Build history of the part. All positions in model axes, mm. Face numbers are marked on the shaded views. Round coordinates to 2 decimals unless told otherwise and drop trailing zeros. Order: outer loops, then holes, each group sorted by start corner. A loop starts at its lowest first (then second) coordinate and runs counter-clockwise, first axis right, second up. Notation, with made-up numbers: (76, 54) -> (118, 54) arc R34 cw to (118, 92) -> close; hole circle Ø8 at (67, 51). An arc over 180 degrees is marked (long way). Answer as a JSON object with one key per item and string values.
from build123d import *

# Parameters (mm, degrees)
BOSS_EXTRUDE1_DEPTH = 4
SKETCH2_R           = 6
BOSS_EXTRUDE2_DEPTH = 1
SKETCH3_R           = 3.95
BOSS_EXTRUDE3_DEPTH = 7
SKETCH4_R           = 2
CUT_EXTRUDE1_DEPTH  = 113.187343315


with BuildPart() as part:
    # Sketch1 → Boss-Extrude1 (new body)
    with BuildSketch(Plane(origin=(0, 0, 0), x_dir=(1, 0, 0), z_dir=(0, 1, 0))):
        with BuildLine():
            Line((0, 11), (100, 11))
            ThreePointArc((100, 11), (111, 0), (100, -11))
            Line((100, -11), (0, -11))
            ThreePointArc((0, -11), (-11, 0), (0, 11))
        make_face()
    extrude(amount=BOSS_EXTRUDE1_DEPTH)

    # Sketch2 → Boss-Extrude2 (add)
    with BuildSketch(Plane(origin=(0, 4, 0), x_dir=(1, 0, 0), z_dir=(0, 1, 0))):
        with Locations(Location((0, 0, 0), (0, 0, 270))):
            Circle(SKETCH2_R)
        with Locations(Location((100, 0, 0), (0, 0, 270))):
            Circle(SKETCH2_R)
    extrude(amount=BOSS_EXTRUDE2_DEPTH)

    # Sketch3 → Boss-Extrude3 (add)
    with BuildSketch(Plane(origin=(0, 5, 0), x_dir=(1, 0, 0), z_dir=(0, 1, 0))):
        with Locations(Location((0, 0, 0), (0, 0, 270))):
            Circle(SKETCH3_R)
        with Locations(Location((100, 0, 0), (0, 0, 270))):
            Circle(SKETCH3_R)
    extrude(amount=BOSS_EXTRUDE3_DEPTH)

    # Sketch4 → Cut-Extrude1 (cut, through all)
    with BuildSketch(Plane(origin=(0, 12, 0), x_dir=(1, 0, 0), z_dir=(0, 1, 0))):
        with Locations(Location((0, 0, 0), (0, 0, 270))):
            Circle(SKETCH4_R)
        with Locations(Location((100, 0, 0), (0, 0, 270))):
            Circle(SKETCH4_R)
    extrude(amount=-CUT_EXTRUDE1_DEPTH, mode=Mode.SUBTRACT)


solid = part.part
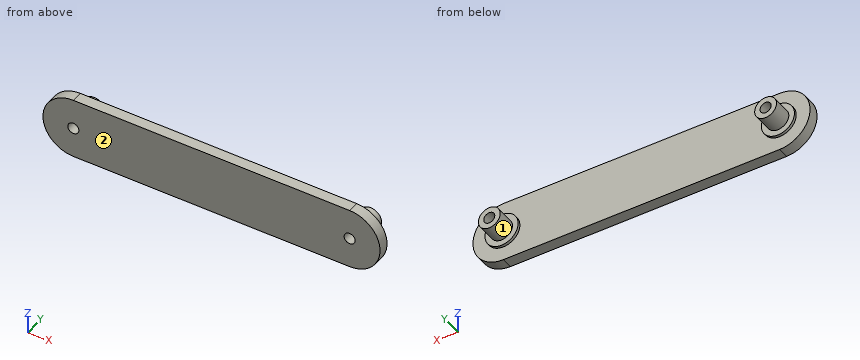
1) Pull direction X, two halves, no side cores. Call the marked faces 1 and 2: pulls with the +X half, pulls with the -X half, needs draft (parallel to the pull), parting line crosses it, or undercut.
Checked values:
{"face 1": "undercut", "face 2": "needs draft"}
2) Cut at C-C, the plane y = 2. Give the cut face in (x, z).
Checked values:
{"outline": "(0, -11) -> (100, -11) arc R11 ccw to (100, 11) -> (0, 11) arc R11 ccw to start; hole circle Ø4 at (0, 0); hole circle Ø4 at (100, 0)"}
3) Flat gauge pins, fed straight in: pin 1 Ø6.5 at (x, z) = (78.5, 4.5) entering from +Y; pin 2 Ø2 at (y, z) = (3.5, -7.5) entering from +X; pin 3 Ø5 at (y, z) = (8.5, -6) entering from -X. Where does each tip first touch, or does it go through?
Checked values:
{"pin 1": "stops at y = 4", "pin 2": "stops at x = 108.87", "pin 3": "stops at x = -1.83"}
4) Cut at A-A, the plane z = 0. Give the cut face in (x, y), plus the area to 3 significant figures.
Checked values:
{"outline": "(-11, 0) -> (-2, 0) -> (-2, 12) -> (-3.95, 12) -> (-3.95, 5) -> (-6, 5) -> (-6, 4) -> (-11, 4) -> close; (2, 0) -> (98, 0) -> (98, 12) -> (96.05, 12) -> (96.05, 5) -> (94, 5) -> (94, 4) -> (6, 4) -> (6, 5) -> (3.95, 5) -> (3.95, 12) -> (2, 12) -> close; (102, 0) -> (111, 0) -> (111, 4) -> (106, 4) -> (106, 5) -> (103.95, 5) -> (103.95, 12) -> (102, 12) -> close", "area": "527 mm²"}
5) Probe L1, parallel to X at y = 3, z = 0; L2, parallel to X at y = 5.75, z = 0; L3, parallel to X at y = 4.75, z = 0. List the from-to ranges inside material, lowest first. Write a range as from..to.
Checked values:
{"L1": "x = -11..-2, 2..98, 102..111", "L2": "x = -3.95..-2, 2..3.95, 96.05..98, 102..103.95", "L3": "x = -6..-2, 2..6, 94..98, 102..106"}
6) Cut at B-B, the plane y = 9. Give the cut face in (x, z).
Checked values:
{"outline": "circle Ø7.9 at (0, 0); circle Ø7.9 at (100, 0); hole circle Ø4 at (0, 0); hole circle Ø4 at (100, 0)"}
7) Cut at D-D, the plane z = 5. Give the cut face in (x, y).
Checked values:
{"outline": "(-9.8, 0) -> (109.8, 0) -> (109.8, 4) -> (103.32, 4) -> (103.32, 5) -> (96.68, 5) -> (96.68, 4) -> (3.32, 4) -> (3.32, 5) -> (-3.32, 5) -> (-3.32, 4) -> (-9.8, 4) -> close"}
